Build history of the part. All positions in model axes, mm. A direction names the side the tool comes from. Coordinates: 2 decimals unless noted, no trailing zeros. Order: outer loops, then holes, each group sorted by start corner. A loop starts at its lowest first (then second) coordinate and runs counter-clockwise, first axis right, second up. Notation, with made-up numbers: (26.25, 62) - (46.25, 62) arc R21 ccw to (46.25, 94) - close; hole circle Ø10 at (22.25, 26.25). An arc over 180 degrees is marked (long way). Return JSON: item names as keys, results as strings.
from build123d import *

# Parameters (mm, degrees)
SKETCH1_R            = 36.83
BOSS_EXTRUDE1_DEPTH  = 31.115
SKETCH2_R            = 24
BOSS_EXTRUDE2_DEPTH  = 4.318
SKETCH5_R            = 2.794
BOSS_EXTRUDE5_DEPTH  = 0.7112
SKETCH14_R           = 15.6337
BOSS_EXTRUDE11_DEPTH = 4.8514
SKETCH15_R           = 12.8016
BOSS_EXTRUDE12_DEPTH = 5.2832
SKETCH16_R           = 2.7686
BOSS_EXTRUDE13_DEPTH = 0.7112
SKETCH17_R           = 8.1534
BOSS_EXTRUDE14_DEPTH = 7.7724
SKETCH18_R           = 15.4432
BOSS_EXTRUDE15_DEPTH = 15.5702
SKETCH19_R           = 13.7414
BOSS_EXTRUDE16_DEPTH = 21.3106
BOSS_EXTRUDE17_DEPTH = 9.144
SKETCH24_R           = 2.4892
BOSS_EXTRUDE18_DEPTH = 1.9812
SKETCH25_R           = 3.2258
BOSS_EXTRUDE19_DEPTH = 3.048
SKETCH27_R           = 4.59774385
BOSS_EXTRUDE20_DEPTH = 26.2382
BOSS_EXTRUDE21_DEPTH = 1.1176


with BuildPart() as part:
    # Sketch1 → Boss-Extrude1 (new body)
    with BuildSketch(Plane.XY):
        with Locations(Location((0, 0, 0), (0, 0, 180))):
            Circle(SKETCH1_R)
    extrude(amount=BOSS_EXTRUDE1_DEPTH)

    # Sketch2 → Boss-Extrude2 (add)
    with BuildSketch(Plane(origin=(0, 0, 0), x_dir=(-1, 0, 0), z_dir=(0, 0, -1))):
        with Locations(Location((0, 0, 0), (0, 0, 180))):
            Circle(SKETCH2_R)
    extrude(amount=BOSS_EXTRUDE2_DEPTH)

    # Sketch5 → Boss-Extrude5 (add)
    with BuildSketch(Plane.XY.offset(31.115)):
        Circle(SKETCH5_R)
    extrude(amount=BOSS_EXTRUDE5_DEPTH)

    # Sketch14 → Boss-Extrude11 (add)
    with BuildSketch(Plane(origin=(0, 0, -4.318), x_dir=(-1, 0, 0), z_dir=(0, 0, -1))):
        Circle(SKETCH14_R)
    extrude(amount=BOSS_EXTRUDE11_DEPTH)

    # Sketch15 → Boss-Extrude12 (add)
    with BuildSketch(Plane(origin=(0, 0, -9.1694), x_dir=(-1, 0, 0), z_dir=(0, 0, -1))):
        Circle(SKETCH15_R)
    extrude(amount=BOSS_EXTRUDE12_DEPTH)

    # Sketch16 → Boss-Extrude13 (add)
    with BuildSketch(Plane(origin=(0, 0, -14.4526), x_dir=(-1, 0, 0), z_dir=(0, 0, -1))):
        Circle(SKETCH16_R)
    extrude(amount=BOSS_EXTRUDE13_DEPTH)



with BuildPart() as body_2:
    # Sketch17 → Boss-Extrude14 (new body)
    with BuildSketch(Plane(origin=(0, 0, -9.1694), x_dir=(-1, 0, 0), z_dir=(0, 0, -1))):
        with Locations((2.110216379, 50.3809)):
            Circle(SKETCH17_R)
    extrude(amount=-BOSS_EXTRUDE14_DEPTH)

    # Sketch18 → Boss-Extrude15 (add)
    with BuildSketch(Plane.XY.offset(-1.397)):
        with Locations((-2.110216379, 50.3809)):
            Circle(SKETCH18_R)
    extrude(amount=BOSS_EXTRUDE15_DEPTH)

    # Sketch19 → Boss-Extrude16 (add)
    with BuildSketch(Plane.XY.offset(14.1732)):
        with Locations((-2.110216379, 50.3809)):
            Circle(SKETCH19_R)
    extrude(amount=BOSS_EXTRUDE16_DEPTH)


with BuildPart() as part_1:
    add(part.part)

    add(body_2.part)  # Boss-Extrude17 merges body 2
    # Sketch23 → Boss-Extrude17 (add)
    with BuildSketch(Plane(origin=(0, 0, -9.1694), x_dir=(-1, 0, 0), z_dir=(0, 0, -1))):
        Polygon((15.6337, 0), (10.263616379, 50.3809), (-6.043183621, 50.3809), (-15.6337, 0), align=None)
    extrude(amount=-BOSS_EXTRUDE17_DEPTH)

    # Sketch24 → Boss-Extrude18 (add)
    with BuildSketch(Plane(origin=(0, 0, -9.1694), x_dir=(-1, 0, 0), z_dir=(0, 0, -1))):
        with Locations((2.110216379, 50.3809)):
            Circle(SKETCH24_R)
    extrude(amount=BOSS_EXTRUDE18_DEPTH)

    # Sketch25 → Boss-Extrude19 (add)
    with BuildSketch(Plane(origin=(0, 0, -9.1694), x_dir=(-1, 0, 0), z_dir=(0, 0, -1))):
        with Locations(Location((1.632950373, 38.986290822, 0), (0, 0, 180))):
            Circle(SKETCH25_R)
    extrude(amount=BOSS_EXTRUDE19_DEPTH)

    # Sketch27 → Boss-Extrude20 (add)
    with BuildSketch(Plane.XY.offset(35.4838)):
        with Locations((15.541092999, 38.356894356)):
            Circle(SKETCH27_R)
    extrude(amount=-BOSS_EXTRUDE20_DEPTH)

    # Sketch29 → Boss-Extrude21 (add)
    with BuildSketch(Plane.XY.offset(35.4838)):
        Polygon((-3.486888815, 64.053165612), (-7.024727103, 68.509088458), (-18.323674319, 59.53814137), (-14.946759387, 55.284902198), align=None)
    extrude(amount=-BOSS_EXTRUDE21_DEPTH)


solid = part_1.part
1. Mould opens along Y. For faces 5 (the cylindrical face through (-2.29, 58.532, -5.338)), 6 (the cylindrical face through (-0.05, -36.83, 15.34)), 7 (the flat face through (0, 3, -14.453)) say: pulls with the +Y half, pulls with the -Y half, needs draft (parallel to the pull), parting line crosses it, or undercut.
Check values:
{"face 5": "pulls with the +Y half", "face 6": "undercut", "face 7": "needs draft"}
2. Tool access for faces 1 (the flat face through (0, 0, 31.826)), 2 (the flat face through (-24, 7, 0)), 3 (the cylindrical face through (-1.79, 52.85, -10.15)), 4 (the flat face through (-5.23, 66.25, 34.93)): list every direction of +Z, -Z, +X, -X, +Y, -Y with a clear straight run to the whole face (end or side of a thin tool).
Check values:
{"face 1": "+Z, +X, -X, -Y", "face 2": "none", "face 3": "-Z", "face 4": "+Z, +X, +Y"}
3. Cut at A-A on y = 0. Give the cut face in (x, z) (3 decimals).
Check values:
{"outline": "(-36.83, 0) - (-24, 0) - (-24, -4.318) - (-15.634, -4.318) - (-15.634, -9.169) - (-12.802, -9.169) - (-12.802, -14.453) - (-2.769, -14.453) - (-2.769, -15.164) - (2.769, -15.164) - (2.769, -14.453) - (12.802, -14.453) - (12.802, -9.169) - (15.634, -9.169) - (15.634, -4.318) - (24, -4.318) - (24, 0) - (36.83, 0) - (36.83, 31.115) - (2.794, 31.115) - (2.794, 31.826) - (-2.794, 31.826) - (-2.794, 31.115) - (-36.83, 31.115) - close"}
4. Cut at D-D on x = 30.5. Give the cut face in (y, z) (3 decimals), plus the area to 3 significant figures.
Check values:
{"outline": "(-20.645, 0) - (20.645, 0) - (20.645, 31.115) - (-20.645, 31.115) - close", "area": "1,280 mm²"}
5. Cut at C-C on y = 46. Give the cut face in (x, z).
Check values:
{"outline": "(-16.92, -1.4) - (-10.73, -1.4) - (-10.73, -9.17) - (6.88, -9.17) - (6.88, -1.4) - (12.7, -1.4) - (12.7, 14.17) - (10.91, 14.17) - (10.91, 35.48) - (-15.13, 35.48) - (-15.13, 14.17) - (-16.92, 14.17) - close"}
6. Probe L1, parallel to Z at x = 2, y = 6 (3 decimals); L2, parallel to Z at x = -29, y = 19.5 (3 decimals); L3, parallel to Y at x = 6.5, z = 28. List the from-to ranges inside material, lowest first.
Check values:
{"L1": "-14.453 to 31.115", "L2": "0 to 31.115", "L3": "-36.25 to 36.25, 39.67 to 61.09"}
7. Drop flat-ended pins along their axis: pin 1 (4.5 mm diameter, centred on x = 14, y = 40, fed in from -Z); pin 2 (12 mm diameter, centred on x = 12.5, z = 25.5, fed in from +Y); pin 3 (15.5 mm diameter, centred on x = -1, y = 14, fed in from -Z). Give the stop position or say it passes through.
Check values:
{"pin 1": "z = 9.25", "pin 2": "y = 61.09", "pin 3": "z = -14.45"}
8. Cut at B-B on z = 29. Give the cut face in (x, y), plus the area to 3 significant figures.
Check values:
{"outline": "(-3.25, 36.69) arc R36.83 ccw (long way) to (14.37, 33.91) arc R4.6 ccw (long way) to (13.29, 34.35) arc R36.83 ccw to (0.17, 36.83) arc R13.74 ccw (long way) to start", "area": "4,920 mm²"}
